Design review of the part built by this model. Coordinates are the model's own, in mm. A direction names the side the tool comes from. Coordinates: 2 decimals unless noted, no trailing zeros. Order: outer loops, then holes, each group sorted by start corner. A loop starts at its lowest first (then second) coordinate and runs counter-clockwise, first axis right, second up. Notation, with made-up numbers: M 47,21.25 L 66,21.25 A28 ccw 66,52.25 Z; hole C 22.5,65.5 d2. An arc over 180 degrees is marked long. Answer as a JSON object with one key per item and string values.
from build123d import *

# Parameters (mm, degrees)
F1_DEPTH       = 15
F3_DEPTH       = 15
F5_D           = 13.2
F5_DEPTH       = 60
F5_CBORE_D     = 19.25
F5_CBORE_DEPTH = 0
F5_TIP         = 3.9656800856
F7_D           = 13.2
F7_DEPTH       = 60
F7_CBORE_D     = 19.25
F7_CBORE_DEPTH = 0
F7_TIP         = 3.9656800856


# Not quite as in the source:
# - ends of sketch curves that miss each other by under 0.0002 mm in the source are joined


with BuildPart() as f1:
    # F0 (on Top) → F1 (new body, symmetric)
    with BuildSketch(Plane.XY):
        with BuildLine():
            Line((-32.5, -15), (-32.5, 15))
            ThreePointArc((-32.5, 15), (-47.5306145724, 0), (-32.5, -15))
        make_face()
        with BuildLine():
            ThreePointArc((-32.5000000638, -14.9999687584), (-21.9131945085, -10.595772326), (-17.5306145724, 0))
            ThreePointArc((-17.5306145724, 0), (-21.9131945085, 10.595772326), (-32.5000000638, 14.9999687584))
            Line((-32.5000000638, 14.9999687584), (-32.5000000638, -14.9999687584))
        make_face()
        with BuildLine():
            ThreePointArc((-32.5000000638, 14.9999687584), (-21.9131945085, 10.595772326), (-17.5306145724, 0))
            ThreePointArc((-17.5306145724, 0), (-21.9131945085, -10.595772326), (-32.5000000638, -14.9999687584))
            Line((-32.5000000638, -14.9999687584), (32.5, -15))
            Line((32.5, -15), (32.5, 15))
            Line((32.5, 15), (-32.5000000638, 14.9999687584))
        make_face()
    extrude(amount=F1_DEPTH, both=True)

    # F2 (on Right) → F3 (cut)
    with BuildSketch(Plane.YZ):
        Polygon((9.5593853593, 5.4426588685), (9.4931735239, -5.5573411315), (-0.0662118354, -11), (17.534378916, -11.1163873225), (17.534378916, 11), (0.0662118354, 11), align=None)
        Polygon((-0.0662118354, -11), (9.4931735239, -5.5573411315), (9.5593853593, 5.4426588685), (0.0662118354, 11), (-9.4931735239, 5.5573411315), (-9.5593853593, -5.4426588685), align=None)
    extrude(amount=-F3_DEPTH, mode=Mode.SUBTRACT)

    # F5
    with Locations(Plane(origin=(0, 0, -15), x_dir=(1, 0, 0), z_dir=(0, 0, -1))):
        with Locations((-32.5306145724, 0)):
            CounterBoreHole(F5_D / 2, F5_CBORE_D / 2, F5_CBORE_DEPTH, depth=F5_DEPTH)
            with Locations((0, 0, -(F5_DEPTH + F5_TIP / 2))):  # 118° drill point
                Cone(0, F5_D / 2, F5_TIP, mode=Mode.SUBTRACT)

    # F7
    with Locations(Plane.YZ.offset(32.5)):
        with Locations((0, 0)):
            CounterBoreHole(F7_D / 2, F7_CBORE_D / 2, F7_CBORE_DEPTH, depth=F7_DEPTH)
            with Locations((0, 0, -(F7_DEPTH + F7_TIP / 2))):  # 118° drill point
                Cone(0, F7_D / 2, F7_TIP, mode=Mode.SUBTRACT)


solid = f1.part
1) Add section D-D (x = -21). State the section outline as (y, z) points.
Taken from the geometry:
{"outline": "M -15,-15 L 15,-15 L 15,15 L -15,15 Z; hole C 0,0 d13.2"}
2) Mouldability with a two-part tool opening along Z and no side actions: class faces 4 (the flat face through (-8, 0, -15)), 5 (the cylindrical face through (-38.627, 2.528, 0.21)), 6 (the flat face through (-8, 0, 15)), 7 (the flat face through (-7, 8, 11)) as released by +Z, released by -Z, zero draft, split by the parting line, or undercut.
Taken from the geometry:
{"face 4": "released by -Z", "face 5": "zero draft", "face 6": "released by +Z", "face 7": "undercut"}
3) To check wall thickness, follow L1, parallel to Y at x = -20, z = 0; L2, parallel to X at y = -4, z = -7; L3, parallel to Z at x = -12.5, y = 13.5. State the ranges of each line that lie inside material, in increasing order.
Taken from the geometry:
{"L1": "y = -15 to -6.6, 6.6 to 15", "L2": "x = -46.99 to -37.78, -27.28 to -15, 0 to 32.5", "L3": "z = -15 to -11.09, 11 to 15"}
4) Add section B-B (y = 1.5). State the section outline as (x, z) points, and give its area (3 significant figures).
Taken from the geometry:
{"outline": "M -47.46,-15 L -38.96,-15 L -38.96,15 L -47.46,15 Z; M -26.1,-15 L 32.5,-15 L 32.5,-6.43 L 0,-6.43 L 0,-11.01 L -15,-11.01 L -15,-6.43 L -26.1,-6.43 Z; M -26.1,6.43 L -15,6.43 L -15,11 L 0,11 L 0,6.43 L 32.5,6.43 L 32.5,15 L -26.1,15 Z", "area": "1,120 mm2"}
5) Insertion check: pin 1 Ø6 at (y, z) = (-2, -0.5) entering from +X. The pin has a flat end and moves straight along its axis. Give the tip position at first contact, or say it passes through.
Taken from the geometry:
{"pin 1": "stops at x = -36.84"}
6) Tool access review of faces 1 (the flat face through (-7.4, -4.88, -8.18)), 2 (the flat face through (0, -15, 0)), 3 (the conical face through (-28.033, -5.712, 0.069)): name each direction out of +Z, -Z, +X, -X, +Y, -Y from which nothing blocks a thin tool from reaching the whole face with its end or side.
Taken from the geometry:
{"face 1": "+Y", "face 2": "+Z, -Z, +X, -X, -Y", "face 3": "+X"}
7) Add section C-C (y = 10.5). State the section outline as (x, z) points.
Taken from the geometry:
{"outline": "M -43.24,-15 L 32.5,-15 L 32.5,15 L -43.24,15 Z; hole M -15,-11.07 L 0,-11.07 L 0,11 L -15,11 Z"}
